from build123d import *

# Parameters (mm, degrees)
F0_W     = 25.4
F0_H     = 25.4
F1_DEPTH = 25.4
F3_DEPTH = 25.401
F4_DEPTH = 25.4010001
F5_DEPTH = 25.4010001
F6_DEPTH = 25.4010001
F7_R     = 3.3987951376
F8_DEPTH = 25.4010001


with BuildPart() as f1:
    # F0 (on Front) → F1 (new body)
    with BuildSketch(Plane.XZ):
        Rectangle(F0_W, F0_H)
    extrude(amount=F1_DEPTH)

    # F2 (on face) → F3 (cut, through all)
    with BuildSketch(Plane.XZ.offset(25.4)):
        with BuildLine():
            add(Edge.make_bspline(
                [(-12.7, 12.7), (-9.1949671809, 8.4666666667), (-2.1849015426, 0), (-9.1949671809, -8.4666666667), (-12.7, -12.7)],
                knots=[0, 0, 0, 0, 0.5, 1, 1, 1, 1], degree=3))
            Line((-12.7, 12.7), (-12.7, -12.7))
        make_face()
    extrude(amount=-F3_DEPTH, mode=Mode.SUBTRACT)

    # F2 (on face) → F4 (cut, through all)
    with BuildSketch(Plane.XZ.offset(25.4)):
        with BuildLine():
            Line((12.7, 12.7), (-12.7, 12.7))
            add(Edge.make_bspline(
                [(-12.7, 12.7), (-8.4666666667, 9.6461512916), (0, 3.5384538747), (8.4666666667, 9.6461512916), (12.7, 12.7)],
                knots=[0, 0, 0, 0, 0.5, 1, 1, 1, 1], degree=3))
        make_face()
    extrude(amount=-F4_DEPTH, mode=Mode.SUBTRACT)

    # F2 (on face) → F5 (cut, through all)
    with BuildSketch(Plane.XZ.offset(25.4)):
        with BuildLine():
            Line((12.7, -12.7), (12.7, 12.7))
            add(Edge.make_bspline(
                [(12.7, 12.7), (9.0947037864, 8.4666666667), (2.2844962136, 0), (9.0947037864, -8.4666666667), (12.7, -12.7)],
                knots=[0, 0, 0, 0, 0.5, 1, 1, 1, 1], degree=3))
        make_face()
    extrude(amount=-F5_DEPTH, mode=Mode.SUBTRACT)

    # F2 (on face) → F6 (cut, through all)
    with BuildSketch(Plane.XZ.offset(25.4)):
        with BuildLine():
            add(Edge.make_bspline(
                [(-12.7, -12.7), (-8.4666666667, -10.1224012509), (0, -3.0855987491), (8.4666666667, -10.1224012509), (12.7, -12.7)],
                knots=[0, 0, 0, 0, 0.5, 1, 1, 1, 1], degree=3))
            Line((-12.7, -12.7), (12.7, -12.7))
        make_face()
    extrude(amount=-F6_DEPTH, mode=Mode.SUBTRACT)

    # F7 (on face) → F8 (cut, through all)
    with BuildSketch(Plane.XZ.offset(25.4)):
        Circle(F7_R)
    extrude(amount=-F8_DEPTH, mode=Mode.SUBTRACT)


solid = f1.part
Geometry: final body of the model. Coordinates: model frame, mm. Give positions to 0.01 mm unless a question says otherwise; leave off trailing zeros. Put each result on its own line as item: value.
Q1. Pin query (flat end, axial travel): pin 1 (12 mm diameter, centred on x = 8, y = -18, fed in from -Z); pin 2 (2 mm diameter, centred on x = 8.5, y = -20, fed in from -Z); pin 3 (4 mm diameter, centred on y = -7, z = 9, fed in from +X). Return the tip coordinate at first contact, or that it passes through.
Here are the results:
pin 1: stops at z = -12.7
pin 2: stops at z = -10.64
pin 3: stops at x = 11.27
Q2. Draft query along Z for faces 1 (the face through (3.242, -12.878, 1.021)), 2 (the face through (-2, 0, 3)). Return one class per face: released by +Z, released by -Z, zero draft, split by the parting line, or undercut.
Here are the results:
face 1: undercut
face 2: zero draft
Q3. Material intervals for L1, parallel to Z at x = 0, y = -8.5; L2, parallel to Z at x = 11.5, y = -14; L3, parallel to X at y = -22, z = -7.75, sorted ascending.
Here are the results:
L1: z = -6.6 to -3.4, 3.4 to 6.59
L2: z = -11.95 to -11.28, 11.28 to 11.84
L3: x = -8.81 to -4.54, 4.54 to 8.77
